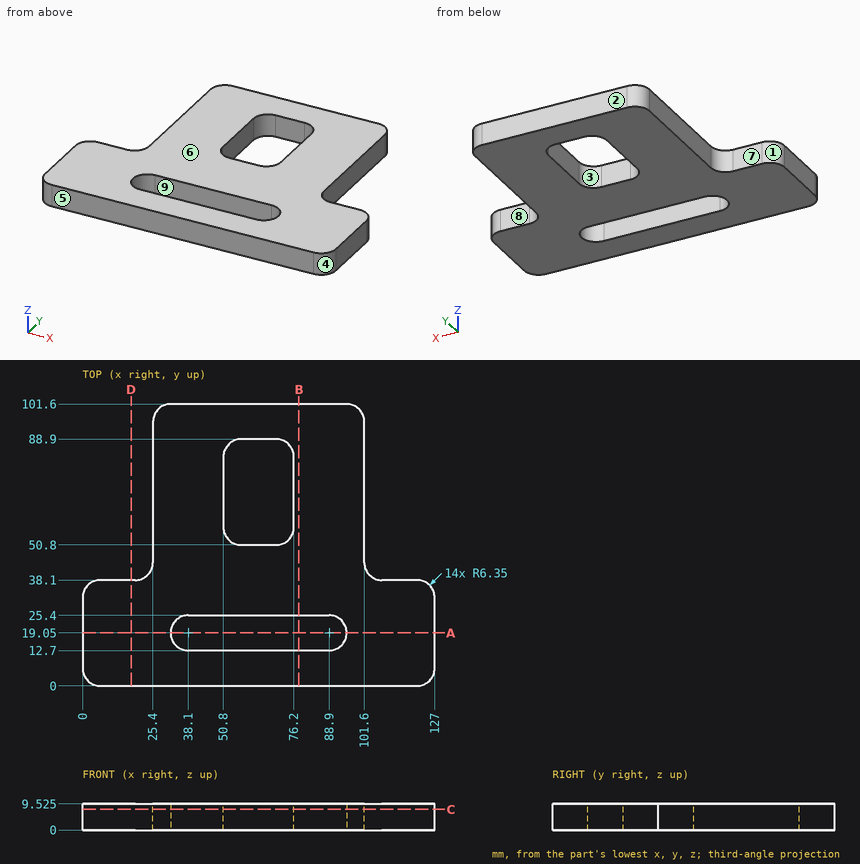
Study the drawing (mm; zero at the part's minimum x, y, z) and answer. A direction names the side the tool comes from. Coordinates: 2 decimals unless noted, no trailing zeros. Write each loop counter-clockwise with the first axis right and the second up, starting at its lowest first coordinate (ties: lowest second). Pieces come first, ordered by that corner, then holes. Notation, with made-up numbers: (4.5, -3) - (23.5, -3) arc R19 cw to (23.5, 34) - close; hole circle Ø10 at (-17, 87). An arc over 180 degrees is marked (long way). Return JSON: item names as keys, results as strings. Group by question number.
1. Determine the mould class of the marked faces 1, 2, 3 and 4 for opening direction X: released by +X, released by -X, zero draft, split by the parting line, or undercut.
2. A cutting plane is placed at D-D, the plane x = 17.5. Determine the outline of the cut face in (y, z) (3 decimals).
3. A cutting plane is placed at B-B, the plane x = 78. Determine the outline of the cut face in (y, z) (3 decimals).
4. A cutting plane is placed at C-C, the plane z = 7.5. Determine the outline of the cut face in (x, y), plus the area to 3 significant figures.
5. Which of the six approach directions +Z, -Z, +X, -X, +Y, -Y give full straight-line access (tool end or side, diameter ignored) to the marked faces 5, 6, 7, 8 and 9?
6. Given pin 1 (3 mm diameter, centred on x = 112.5, z = 7, fed in from +Y); pin 2 (3 mm diameter, centred on y = 59, z = 4.5, fed in from +X); pin 3 (5 mm diameter, centred on x = 61, z = 1, fed in from -Y); pin 4 (5 mm diameter, centred on y = 64, z = 6, fed in from -X), each flat-ended and moving along its own axis, determine where each tip first touches the part or whether it passes through.
7. A cutting plane is placed at A-A, the plane y = 19.05. Determine the outline of the cut face in (x, z) (3 decimals).
8. Straight lines are drawn through the part: L1, parallel to Y at x = 58.5, z = 1.75; L2, parallel to X at y = 57.5, z = 6.5; L3, parallel to Y at x = 46, z = 7. For each, find the intervals that lie inside material, in ascending order.
Ans:
{
 "1": {"face 1": "released by -X", "face 2": "zero draft", "face 3": "undercut", "face 4": "released by +X"},
 "2": {"outline": "(0, 0) - (38.1, 0) - (38.1, 9.525) - (0, 9.525) - close"},
 "3": {"outline": "(0, 0) - (12.7, 0) - (12.7, 9.525) - (0, 9.525) - close; (25.4, 0) - (101.6, 0) - (101.6, 9.525) - (25.4, 9.525) - close"},
 "4": {"outline": "(0, 6.35) arc R6.35 ccw to (6.35, 0) - (120.65, 0) arc R6.35 ccw to (127, 6.35) - (127, 31.75) arc R6.35 ccw to (120.65, 38.1) - (107.95, 38.1) arc R6.35 cw to (101.6, 44.45) - (101.6, 95.25) arc R6.35 ccw to (95.25, 101.6) - (31.75, 101.6) arc R6.35 ccw to (25.4, 95.25) - (25.4, 44.45) arc R6.35 cw to (19.05, 38.1) - (6.35, 38.1) arc R6.35 ccw to (0, 31.75) - close; hole (38.1, 12.7) - (88.9, 12.7) arc R6.35 ccw to (88.9, 25.4) - (38.1, 25.4) arc R6.35 ccw to start; hole (50.8, 57.15) arc R6.35 ccw to (57.15, 50.8) - (69.85, 50.8) arc R6.35 ccw to (76.2, 57.15) - (76.2, 82.55) arc R6.35 ccw to (69.85, 88.9) - (57.15, 88.9) arc R6.35 ccw to (50.8, 82.55) - close", "area": "7,940 mm²"},
 "5": {"face 5": "+Z, -Z, +X, -X, -Y", "face 6": "+Z, +X, -X, +Y, -Y", "face 7": "+Z, -Z, -X, +Y", "face 8": "+Z, -Z, +X, +Y", "face 9": "+Z, -Z"},
 "6": {"pin 1": "y = 38.1", "pin 2": "x = 101.6", "pin 3": "y = 0", "pin 4": "x = 25.4"},
 "7": {"outline": "(0, 0) - (31.75, 0) - (31.75, 9.525) - (0, 9.525) - close; (95.25, 0) - (127, 0) - (127, 9.525) - (95.25, 9.525) - close"},
 "8": {"L1": "0 to 12.7, 25.4 to 50.8, 88.9 to 101.6", "L2": "25.4 to 50.8, 76.2 to 101.6", "L3": "0 to 12.7, 25.4 to 101.6"}
}
